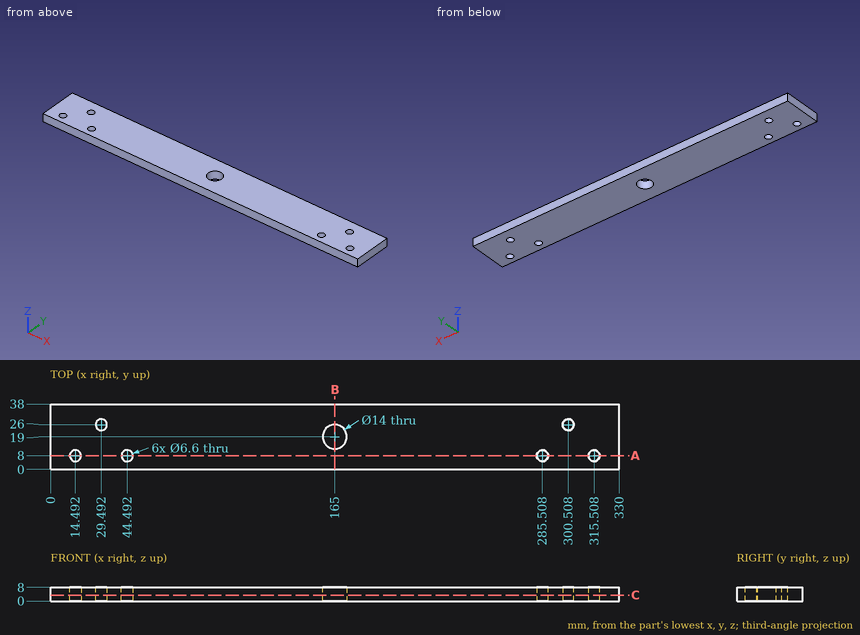
For this review, use the dimensioned drawing (mm, ordinates from the lowest corner) and the shaded views. Round coordinates to 2 decimals unless told otherwise and drop trailing zeros. Order: outer loops, then holes, each group sorted by start corner. A loop starts at its lowest first (then second) coordinate and runs counter-clockwise, first axis right, second up. Notation, with made-up numbers: (19, 3.5) -> (50, 3.5) arc R9 cw to (50, 7.5) -> close; hole circle Ø2 at (11.25, 63). An arc over 180 degrees is marked (long way). One line per item, written item: value. Start each with the question number.
Q1. Take a section at A-A (y = 8). Write out the cut boundary in (x, z).
Q2. Clearance check with a flat-ended pin moving along its axis: pin 1 Ø12.5 at (x, y) = (165, 19) entering from +Z. State where the tip first meets the part, or that it passes through.
Q3. Take a section at C-C (z = 3.5). Write out the cut boundary in (x, y).
Q4. Wall thickness on line 1 (X direction, y = 26.5, z = 2.25); line 2 (Y direction, x = 44, z = 7.75); line 3 (Y direction, x = 301, z = 4.25): over which ranges is each line inside the solid? List them lowest first.
Q5. Take a section at B-B (x = 165). Write out the cut boundary in (y, z), and give its area (3 significant figures).
Reported:
1. outline: (0, 0) -> (11.19, 0) -> (11.19, 8) -> (0, 8) -> close; (17.79, 0) -> (41.19, 0) -> (41.19, 8) -> (17.79, 8) -> close; (47.79, 0) -> (282.21, 0) -> (282.21, 8) -> (47.79, 8) -> close; (288.81, 0) -> (312.21, 0) -> (312.21, 8) -> (288.81, 8) -> close; (318.81, 0) -> (330, 0) -> (330, 8) -> (318.81, 8) -> close
2. pin 1: passes through
3. outline: (0, 0) -> (330, 0) -> (330, 38) -> (0, 38) -> close; hole circle Ø6.6 at (14.49, 8); hole circle Ø6.6 at (29.49, 26); hole circle Ø6.6 at (44.49, 8); hole circle Ø14 at (165, 19); hole circle Ø6.6 at (285.51, 8); hole circle Ø6.6 at (300.51, 26); hole circle Ø6.6 at (315.51, 8)
4. line 1: x = 0 to 26.23, 32.75 to 297.25, 303.77 to 330
4. line 2: y = 0 to 4.74, 11.26 to 38
4. line 3: y = 0 to 22.74, 29.26 to 38
5. outline: (0, 0) -> (12, 0) -> (12, 8) -> (0, 8) -> close; (26, 0) -> (38, 0) -> (38, 8) -> (26, 8) -> close
5. area: 192 mm2
